The figure shows three views and two pictorial views of one solid part (mm, origin at its lowest corner). Answer the questions. A direction names the side the tool comes from. Round coordinates to 2 decimals unless told otherwise and drop trailing zeros. Loops run counter-clockwise (first coordinate to the right, second up) from the corner with the lowest first, then second, coordinate; pieces in that order, holes last. Notation, with made-up numbers: (52.25, -31.5) -> (94.25, -31.5) arc R17 ccw to (94.25, -24.5) -> close; hole circle Ø6 at (24.5, -15). An arc over 180 degrees is marked (long way). Use a Markdown table: item, result. Add a question column.
Q1. Section C-C on x = 25 is taken. Give the vertices of the cut face in (y, z), then the cut area to 3 significant figures.
Q2. Given pin 1 Ø14.5 at (x, z) = (34, 29.5) entering from +Y; pin 2 Ø6 at (x, z) = (10, 39) entering from -Y; pin 3 Ø5 at (x, y) = (42.5, 28) entering from -Z, each flat-ended and moving along its own axis, determine where each tip first touches the part or whether it passes through.
Q3. Consider line 1 (X direction, y = 0.75, z = 39); line 2 (Y direction, x = 25, z = 49.35); line 3 (Y direction, x = 7.5, z = 49). Determine where each line is inside the solid, lowest interval first.
Q4. Section A-A on y = 40 is taken. Give the vertices of the cut face in (x, z), then the cut area to 3 significant figures.
Q5. Section B-B on z = 9 is taken. Give the vertices of the cut face in (x, y).
Q6. Which of the six approach directions +Z, -Z, +X, -X, +Y, -Y give full straight-line access (tool end or side, diameter ignored) to the marked faces 1 and 2?
Q7. Section D-D on z = 24 is taken. Give the vertices of the cut face in (x, y).
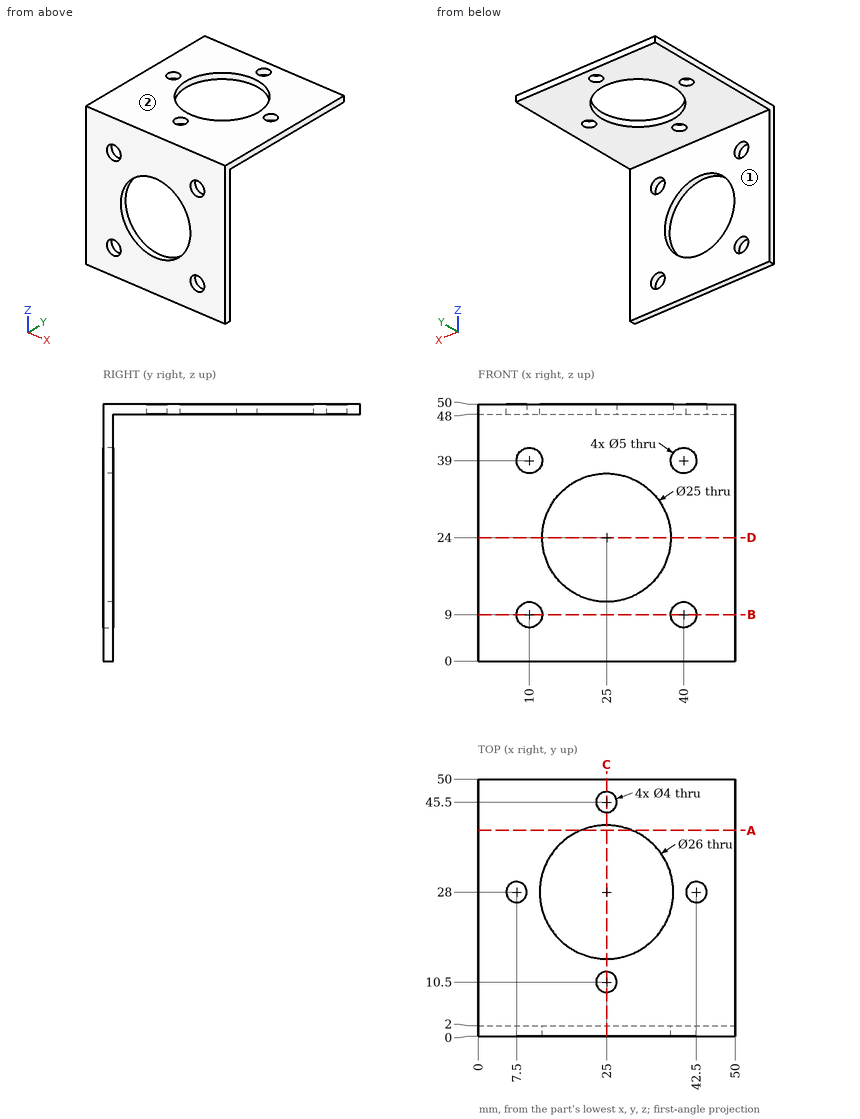
Checked values:
| question | item | result |
|---|---|---|
| 1 | outline | (0, 0) -> (2, 0) -> (2, 11.5) -> (0, 11.5) -> close; (0, 36.5) -> (2, 36.5) -> (2, 48) -> (8.5, 48) -> (8.5, 50) -> (0, 50) -> close; (12.5, 48) -> (15, 48) -> (15, 50) -> (12.5, 50) -> close; (41, 48) -> (43.5, 48) -> (43.5, 50) -> (41, 50) -> close; (47.5, 48) -> (50, 48) -> (50, 50) -> (47.5, 50) -> close |
| 1 | area | 78.0 mm2 |
| 2 | pin 1 | stops at y = 2 |
| 2 | pin 2 | stops at y = 0 |
| 2 | pin 3 | stops at z = 48 |
| 3 | line 1 | x = 0 to 7.5, 12.5 to 37.5, 42.5 to 50 |
| 3 | line 2 | y = 0 to 8.5, 12.5 to 15, 41 to 43.5, 47.5 to 50 |
| 3 | line 3 | y = 0 to 26, 30 to 50 |
| 4 | outline | (0, 48) -> (20, 48) -> (20, 50) -> (0, 50) -> close; (30, 48) -> (50, 48) -> (50, 50) -> (30, 50) -> close |
| 4 | area | 80.0 mm2 |
| 5 | outline | (0, 0) -> (7.5, 0) -> (7.5, 2) -> (0, 2) -> close; (12.5, 0) -> (37.5, 0) -> (37.5, 2) -> (12.5, 2) -> close; (42.5, 0) -> (50, 0) -> (50, 2) -> (42.5, 2) -> close |
| 6 | face 1 | -Z, +X, -X, +Y |
| 6 | face 2 | +Z, +X, -X, +Y, -Y |
| 7 | outline | (0, 0) -> (12.5, 0) -> (12.5, 2) -> (0, 2) -> close; (37.5, 0) -> (50, 0) -> (50, 2) -> (37.5, 2) -> close |
